The listing builds one solid part. Answer for the finished solid, in the listing's coordinates (mm). Face numbers are marked on the shaded views. A direction names the side the tool comes from. Coordinates: 2 decimals unless noted, no trailing zeros. Order: outer loops, then holes, each group sorted by start corner. A loop starts at its lowest first (then second) coordinate and runs counter-clockwise, first axis right, second up. Notation, with made-up numbers: (11, 40.25) - (23, 40.25) arc R24 ccw to (23, 61.25) - close; hole circle Ø5 at (1, -14.75). An arc over 180 degrees is marked (long way). Use a Markdown table: item, result. Add a question column.
Item 1: The part is cut by section A-A, the plane x = 0. Give the vertices of the cut face in (y, z).
Item 2: Flat-ended cylindrical pins translate along their axes: P1, Ø1.3, axis at y = -10.5, z = 3, coming from the -X side; P2, Ø0.9, axis at x = 0, y = 8, coming from the -Z side; P3, Ø0.5, axis at y = 11.5, z = 2.5, coming from the +X side. Find the tip coordinate at first contact, or state that the pin passes through.
Item 3: For the marked faces 1 and 2, determine the directions among +Z, -Z, +X, -X, +Y, -Y from which every point of the face is accessible in a straight line to the end or side of a thin tool.
Item 4: The part is cut by section D-D, the plane y = 6.5. Give the vertices of the cut face in (x, z), then the cut area to 3 significant figures.
Item 5: The part is cut by section C-C, the plane z = 2.75. Give the vertices of the cut face in (x, y).
Item 6: The mould has two halves that part along X. Classify the marked faces 3 and 4: released by +X, released by -X, zero draft, split by the parting line, or undercut.
Item 7: Find the intervals of material crossed by line 1 along X through (y, z) = (20, 2.95); line 2 along Y through (x, z) = (1.25, 5.5); line 3 along Y through (x, z) = (0, 2.7), in increasing order.
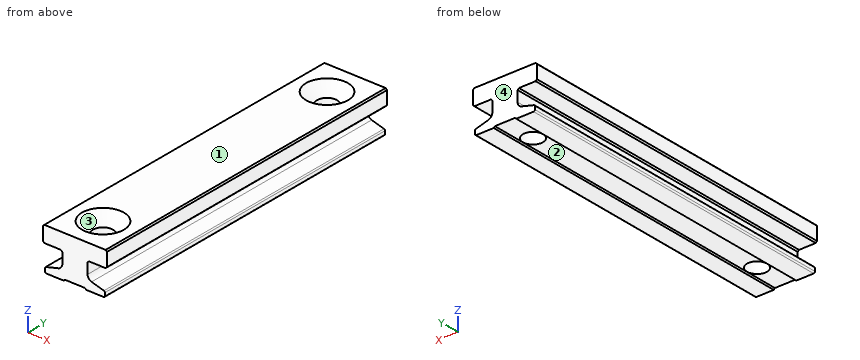
from build123d import *

# Parameters (mm, degrees)
ESQUISSE1_W                                    = 9
ESQUISSE1_H                                    = 50
BOSS_EXTRU_1_DEPTH                             = 6.3
ESQUISSE2_W                                    = 2.6
ESQUISSE2_H                                    = 5.499999997
ENL_V_MAT_EXTRU_1_DEPTH                        = 51.595849632
ESQUISSE3_W                                    = 2.4
ESQUISSE3_H                                    = 50
BOSS_EXTRU_2_DEPTH                             = 2.9
ESQUISSE4_W                                    = 2.6
ESQUISSE4_H                                    = 4.803332101
ENL_V_MAT_EXTRU_2_DEPTH                        = 51.623413555
ESQUISSE5_W                                    = 2.4
ESQUISSE5_H                                    = 50
BOSS_EXTRU_3_DEPTH                             = 2.9
ESQUISSE6_W                                    = 3.04
ESQUISSE6_H                                    = 0.18
ENL_V_MAT_EXTRU_3_DEPTH                        = 51.623413555
D_POUILLE1_ANGLE                               = 14.999999904
D_POUILLE2_ANGLE                               = 14.999999904
D_POUILLE3_ANGLE                               = 45
FRAISAGE_POUR_VIS_T_TE_FRAIS_E_M31_D           = 3
FRAISAGE_POUR_VIS_T_TE_FRAIS_E_M31_CSINK_D     = 6.3
FRAISAGE_POUR_VIS_T_TE_FRAIS_E_M31_CSINK_ANGLE = 90
CHANFREIN1_SIZE                                = 0.2
CONG_1_R                                       = 0.2
CONG_2_R                                       = 0.8


with BuildPart() as part:
    # Esquisse1 → Boss.-Extru.1 (new body)
    with BuildSketch(Plane.XY.offset(6.3)):
        Rectangle(ESQUISSE1_W, ESQUISSE1_H)
    extrude(amount=-BOSS_EXTRU_1_DEPTH)

    # Esquisse2 → Enlèv. mat.-Extru.1 (cut, through all)
    with BuildSketch(Plane(origin=(0, 25, 0), x_dir=(-1, 0, 0), z_dir=(0, 1, 0))):
        with Locations((3.2, 3.550000002)):
            Rectangle(ESQUISSE2_W, ESQUISSE2_H)
    extrude(amount=-ENL_V_MAT_EXTRU_1_DEPTH, mode=Mode.SUBTRACT)

    # Esquisse3 → Boss.-Extru.2 (add)
    with BuildSketch(Plane.ZY.offset(1.9)):
        with Locations((5.1, 0)):
            Rectangle(ESQUISSE3_W, ESQUISSE3_H)
    extrude(amount=BOSS_EXTRU_2_DEPTH)

    # Esquisse4 → Enlèv. mat.-Extru.2 (cut, through all)
    with BuildSketch(Plane(origin=(0, 25, 0), x_dir=(-1, 0, 0), z_dir=(0, 1, 0))):
        with Locations((-3.2, 3.89833395)):
            Rectangle(ESQUISSE4_W, ESQUISSE4_H)
    extrude(amount=-ENL_V_MAT_EXTRU_2_DEPTH, mode=Mode.SUBTRACT)

    # Esquisse5 → Boss.-Extru.3 (add)
    with BuildSketch(Plane(origin=(1.9, 0, 0), x_dir=(0, 0, -1), z_dir=(1, 0, 0))):
        with Locations((-5.1, 0)):
            Rectangle(ESQUISSE5_W, ESQUISSE5_H)
    extrude(amount=BOSS_EXTRU_3_DEPTH)

    # Esquisse6 → Enlèv. mat.-Extru.3 (cut, through all)
    with BuildSketch(Plane.XZ.offset(25)):
        with Locations((0, 0.09)):
            Rectangle(ESQUISSE6_W, ESQUISSE6_H)
    extrude(amount=-ENL_V_MAT_EXTRU_3_DEPTH, mode=Mode.SUBTRACT)

    # Dépouille1
    d_pouille1_faces = [part.faces().sort_by_distance(p)[0] for p in [
        (-3.2, 0, 0.800000003),
    ]]
    draft(d_pouille1_faces, Plane(origin=(-4.5, 25, 0), x_dir=(0, -1, 0), z_dir=(-1, 0, 0)), D_POUILLE1_ANGLE)

    # Dépouille2
    d_pouille2_faces = [part.faces().sort_by_distance(p)[0] for p in [
        (3.2, 0, 1.496667899),
    ]]
    draft(d_pouille2_faces, Plane(origin=(1.9, -25, 1.496667899), x_dir=(0, 0, 1), z_dir=(1, 0, 0)), D_POUILLE2_ANGLE)

    # Dépouille3
    d_pouille3_faces = [part.faces().sort_by_distance(p)[0] for p in [
        (-1.52, 0, 0.09),
        (1.52, 0, 0.09),
    ]]
    draft(d_pouille3_faces, Plane(origin=(1.52, 25, 0.18), x_dir=(-1, 0, 0), z_dir=(0, 0, -1)), D_POUILLE3_ANGLE)

    # Fraisage pour vis à tête fraisée M31 (through all)
    with Locations(Plane.XY.offset(6.3)):
        with Locations((0, 20), (0, -20)):
            CounterSinkHole(FRAISAGE_POUR_VIS_T_TE_FRAIS_E_M31_D / 2, FRAISAGE_POUR_VIS_T_TE_FRAIS_E_M31_CSINK_D / 2, counter_sink_angle=FRAISAGE_POUR_VIS_T_TE_FRAIS_E_M31_CSINK_ANGLE)

    # Chanfrein1
    chanfrein1_edges = [part.edges().sort_by_distance(p)[0] for p in [
        (-1.9, 0, 3.9),
        (-4.8, 0, 6.3),
        (-4.8, 0, 3.9),
        (1.9, 0, 3.9),
        (4.8, 0, 3.9),
        (4.8, 0, 6.3),
    ]]
    chamfer(chanfrein1_edges, length=CHANFREIN1_SIZE)

    # Congé1
    cong_1_edges = [part.edges().sort_by_distance(p)[0] for p in [
        (-4.5, 0, 0),
        (-4.5, 0, 0.800000003),
        (4.5, 0, 0),
        (4.5, 0, 0.800000003),
    ]]
    fillet(cong_1_edges, radius=CONG_1_R)

    # Congé2
    cong_2_edges = [part.edges().sort_by_distance(p)[0] for p in [
        (-1.9, 0, 1.496667899),
        (1.9, 0, 1.496667899),
    ]]
    fillet(cong_2_edges, radius=CONG_2_R)


solid = part.part
Solution:
| question | item | result |
|---|---|---|
| 1 | outline | (-25, 0.18) - (-21.5, 0.18) - (-21.5, 4.65) - (-23.15, 6.3) - (-25, 6.3) - close; (-18.5, 0.18) - (18.5, 0.18) - (18.5, 4.65) - (16.85, 6.3) - (-16.85, 6.3) - (-18.5, 4.65) - close; (21.5, 0.18) - (25, 0.18) - (25, 6.3) - (23.15, 6.3) - (21.5, 4.65) - close |
| 2 | P1 | stops at x = -1.9 |
| 2 | P2 | stops at z = 0.18 |
| 2 | P3 | stops at x = 1.9 |
| 3 | face 1 | +Z, +X, -X, +Y, -Y |
| 3 | face 2 | -Z, +Y, -Y |
| 4 | outline | (-4.8, 4.1) - (-4.6, 3.9) - (-2.1, 3.9) - (-1.9, 3.7) - (-1.9, 2.11) arc R0.8 cw to (-2.49, 1.34) - (-4.35, 0.84) arc R0.2 ccw to (-4.5, 0.65) - (-4.5, 0.2) arc R0.2 ccw to (-4.3, 0) - (-1.7, 0) - (-1.52, 0.18) - (1.52, 0.18) - (1.7, 0) - (4.3, 0) arc R0.2 ccw to (4.5, 0.2) - (4.5, 0.65) arc R0.2 ccw to (4.35, 0.84) - (2.49, 1.34) arc R0.8 cw to (1.9, 2.11) - (1.9, 3.7) - (2.1, 3.9) - (4.6, 3.9) - (4.8, 4.1) - (4.8, 6.1) - (4.6, 6.3) - (-4.6, 6.3) - (-4.8, 6.1) - close |
| 4 | area | 43.3 mm2 |
| 5 | outline | (-1.9, -25) - (1.9, -25) - (1.9, 25) - (-1.9, 25) - close; hole circle Ø3 at (0, -20); hole circle Ø3 at (0, 20) |
| 6 | face 3 | undercut |
| 6 | face 4 | zero draft |
| 7 | line 1 | x = -1.9 to -1.5, 1.5 to 1.9 |
| 7 | line 2 | y = -25 to -21.99, -18.01 to 18.01, 21.99 to 25 |
| 7 | line 3 | y = -25 to -21.5, -18.5 to 18.5, 21.5 to 25 |
